from build123d import *

# Parameters (mm, degrees)
F0_R     = 250
F0_R_2   = 200
F1_DEPTH = 15
F2_R     = 7.5
F3_DEPTH = 15
F5_R     = 200
F5_R_2   = 195
F6_DEPTH = 5


with BuildPart() as f1:
    # F0 (on Top) → F1 (new body)
    with BuildSketch(Plane.XY):
        Circle(F0_R)
        Circle(F0_R_2, mode=Mode.SUBTRACT)
    extrude(amount=F1_DEPTH)

    # F2 (on face) → F3 (cut, through all)
    with BuildSketch(Plane.XY.offset(15)):
        with Locations((227.5, 0)):
            Circle(F2_R)
        with Locations((197.020779, 113.75)):
            Circle(F2_R)
        with Locations((113.75, 197.020779)):
            Circle(F2_R)
        with Locations((0, 227.5)):
            Circle(F2_R)
        with Locations((-113.75, 197.020779)):
            Circle(F2_R)
        with Locations((-197.020779, 113.75)):
            Circle(F2_R)
        with Locations((-227.5, 0)):
            Circle(F2_R)
        with Locations((-197.020779, -113.75)):
            Circle(F2_R)
        with Locations((-113.75, -197.020779)):
            Circle(F2_R)
        with Locations((0, -227.5)):
            Circle(F2_R)
        with Locations((113.75, -197.020779)):
            Circle(F2_R)
        with Locations((197.020779, -113.75)):
            Circle(F2_R)
    extrude(amount=-F3_DEPTH, mode=Mode.SUBTRACT)

    # F5 (on offset) → F6 (join)
    with BuildSketch(Plane.XY.offset(5)):
        Circle(F5_R)
        Circle(F5_R_2, mode=Mode.SUBTRACT)
    extrude(amount=F6_DEPTH)


solid = f1.part
Verification items for the finished model (mm, model axes). A direction names the side the tool comes from. Coordinates: 2 decimals unless noted, no trailing zeros. Write each loop counter-clockwise with the first axis right and the second up, starting at its lowest first coordinate (ties: lowest second). Pieces come first, ordered by that corner, then holes. Notation, with made-up numbers: M 5,21 L 28,21 A3 ccw 28,26 Z; hole C 12.5,-32.5 d7. An arc over 180 degrees is marked long. Use CSV: the item, a comma, the result in double quotes.
Q1. Thickness scan on line 1 along Y through (x, z) = (0, 3); line 2 along Y through (x, z) = (-227.5, 6.5); line 3 along X through (y, z) = (-79, 1.5). Record the ranges inside material, lowest first. Write a range as [from, to].
Computed values:
line 1,"[-250, -235], [-220, -200], [200, 220], [235, 250]"
line 2,"[-103.65, -7.5], [7.5, 103.65]"
line 3,"[-237.19, -183.74], [183.74, 237.19]"
Q2. Set-up check for faces 1 (the flat face through (192, -44, 5)), 2 (the cylindrical face through (-0.976, -220.064, 7.605)), 3 (the cylindrical face through (190.764, 60.075, 12.465)): record each of +Z, -Z, +X, -X, +Y, -Y from which the full face is reachable in a straight line by a thin tool's end or side.
Computed values:
face 1,"-Z"
face 2,"+Z, -Z"
face 3,"+Z"
Q3. Section check C-C, the plane y = 80.5. Enter the section's corners in (x, z).
Computed values:
outline,"M -236.68,0 L -183.08,0 L -183.08,5 L -177.61,5 L -177.61,10 L -183.08,10 L -183.08,15 L -236.68,15 Z; M 177.61,5 L 183.08,5 L 183.08,0 L 236.68,0 L 236.68,15 L 183.08,15 L 183.08,10 L 177.61,10 Z"
Q4. Section check A-A, the plane y = 0. Enter the section's corners in (x, z), and give its area (3 significant figures).
Computed values:
outline,"M -250,0 L -235,0 L -235,15 L -250,15 Z; M -220,0 L -200,0 L -200,5 L -195,5 L -195,10 L -200,10 L -200,15 L -220,15 Z; M 195,5 L 200,5 L 200,0 L 220,0 L 220,15 L 200,15 L 200,10 L 195,10 Z; M 235,0 L 250,0 L 250,15 L 235,15 Z"
area,"1,100 mm²"
Q5. Go/stop test with flat-tipped pins: P1, Ø3, axis at x = -51.5, z = 6, coming from the +Y side; P2, Ø6, axis at x = 152.5, z = 10.5, coming from the +Y side; P3, Ø1.5, axis at x = -81, z = 7, coming from the -Y side. Record where each tip stops, or that it passes through.
Computed values:
P1,"y = 244.95"
P2,"y = 200.37"
P3,"y = -236.77"
Q6. Section check D-D, the plane x = -149. Enter the section's corners in (y, z), and give its area (3 significant figures).
Computed values:
outline,"M -200.75,0 L -133.41,0 L -133.41,5 L -125.79,5 L -125.79,10 L -133.41,10 L -133.41,15 L -200.75,15 Z; M 125.79,5 L 133.41,5 L 133.41,0 L 200.75,0 L 200.75,15 L 133.41,15 L 133.41,10 L 125.79,10 Z"
area,"2,100 mm²"
Q7. Mould release check, pull along X, two halves, no side actions. Record for faces 4 (the cylindrical face through (-249.76, 10.99, 7.4)), 5 (the cylindrical face through (195.39, 106.43, 7.6)), 6 (the flat face through (-75, 186, 0)): pulls with the +X half, pulls with the -X half, needs draft (parallel to the pull), parting line crosses it, or undercut.
Computed values:
face 4,"parting line crosses it"
face 5,"undercut"
face 6,"needs draft"
